from build123d import *

# Parameters (mm, degrees)
CYLINDER032_R     = 2
CYLINDER032_DEPTH = 8
CYLINDER035_R     = 2
CYLINDER035_DEPTH = 8
CYLINDER038_R     = 1.6
CYLINDER038_DEPTH = 8
CYLINDER039_R     = 1.6
CYLINDER039_DEPTH = 8
CYLINDER037_W     = 7
CYLINDER037_H     = 8
CYLINDER037_ANGLE = 90
BOX025_W          = 78
BOX025_H          = 3
BOX025_DEPTH      = 7
BOX026_W          = 40
BOX026_H          = 3
BOX026_DEPTH      = 7
CYLINDER034_R     = 5
CYLINDER034_DEPTH = 8
CYLINDER031_R     = 5
CYLINDER031_DEPTH = 8
BOX027_W          = 40
BOX027_H          = 3
BOX027_DEPTH      = 7
CYLINDER036_W     = 7
CYLINDER036_H     = 8
CYLINDER036_ANGLE = 90


with BuildPart() as cuts:
    # Cylinder032 → Cylinder032 (new body)
    with BuildSketch(Plane(origin=(13.5, -2, 61.5), x_dir=(1, 0, 0), z_dir=(0, -1, 0))):
        Circle(CYLINDER032_R)
    extrude(amount=CYLINDER032_DEPTH)


with BuildPart() as cuts001:
    # Cylinder035 → Cylinder035 (new body)
    with BuildSketch(Plane(origin=(62.5, -2, 61.5), x_dir=(1, 0, 0), z_dir=(0, -1, 0))):
        Circle(CYLINDER035_R)
    extrude(amount=CYLINDER035_DEPTH)


with BuildPart() as m3screw:
    # Cylinder038 → Cylinder038 (new body)
    with BuildSketch(Plane(origin=(75.5, -2, 100.5), x_dir=(1, 0, 0), z_dir=(0, -1, 0))):
        Circle(CYLINDER038_R)
    extrude(amount=CYLINDER038_DEPTH)


with BuildPart() as c4oldcuts:
    # Cylinder039 → Cylinder039 (new body)
    with BuildSketch(Plane(origin=(2.5, -2, 100.5), x_dir=(1, 0, 0), z_dir=(0, -1, 0))):
        Circle(CYLINDER039_R)
    extrude(amount=CYLINDER039_DEPTH)

    # Fusion016: union cuts, cuts001, m3Screw
    add(cuts.part)
    add(cuts001.part)
    add(m3screw.part)


with BuildPart() as cylinder037:
    # Cylinder037 → Cylinder037 (revolve)
    with BuildSketch(Plane(origin=(0, -2, 98), x_dir=(1, 0, 0), z_dir=(0, 0, -1))):
        with Locations((3.5, 4)):
            Rectangle(CYLINDER037_W, CYLINDER037_H)
    revolve(axis=Axis((0, -2, 98), (0, -1, 0)), revolution_arc=CYLINDER037_ANGLE)


with BuildPart() as cube020:
    # Box025 → Box025 (new body)
    with BuildSketch(Plane(origin=(0, -5, 58), x_dir=(1, 0, 0), z_dir=(0, 0, 1))):
        with Locations((39, 1.5)):
            Rectangle(BOX025_W, BOX025_H)
    extrude(amount=BOX025_DEPTH)


with BuildPart() as cube021:
    # Box026 → Box026 (new body)
    with BuildSketch(Plane(origin=(7, -5, 58), x_dir=(0, 0, 1), z_dir=(-1, 0, 0))):
        with Locations((20, 1.5)):
            Rectangle(BOX026_W, BOX026_H)
    extrude(amount=BOX026_DEPTH)


with BuildPart() as cylinder034:
    # Cylinder034 → Cylinder034 (new body)
    with BuildSketch(Plane(origin=(62.5, -2, 61.5), x_dir=(1, 0, 0), z_dir=(0, -1, 0))):
        Circle(CYLINDER034_R)
    extrude(amount=CYLINDER034_DEPTH)


with BuildPart() as cylinder031:
    # Cylinder031 → Cylinder031 (new body)
    with BuildSketch(Plane(origin=(13.5, -2, 61.5), x_dir=(1, 0, 0), z_dir=(0, -1, 0))):
        Circle(CYLINDER031_R)
    extrude(amount=CYLINDER031_DEPTH)


with BuildPart() as fusion014:
    # Box027 → Box027 (new body)
    with BuildSketch(Plane(origin=(78, -5, 58), x_dir=(0, 0, 1), z_dir=(-1, 0, 0))):
        with Locations((20, 1.5)):
            Rectangle(BOX027_W, BOX027_H)
    extrude(amount=BOX027_DEPTH)

    # Fusion014: union Cube020, Cube021, Cylinder034, Cylinder031
    add(cube020.part)
    add(cube021.part)
    add(cylinder034.part)
    add(cylinder031.part)


with BuildPart() as c4hold001:
    # Cylinder036 → Cylinder036 (revolve)
    with BuildSketch(Plane(origin=(78, -2, 98), x_dir=(0, 0, 1), z_dir=(1, 0, 0))):
        with Locations((3.5, 4)):
            Rectangle(CYLINDER036_W, CYLINDER036_H)
    revolve(axis=Axis((78, -2, 98), (0, -1, 0)), revolution_arc=CYLINDER036_ANGLE)

    # Fusion015: union Cylinder037, Fusion014
    add(cylinder037.part)
    add(fusion014.part)

    # Cut024: cut c4oldCuts
    add(c4oldcuts.part, mode=Mode.SUBTRACT)


solid = c4hold001.part
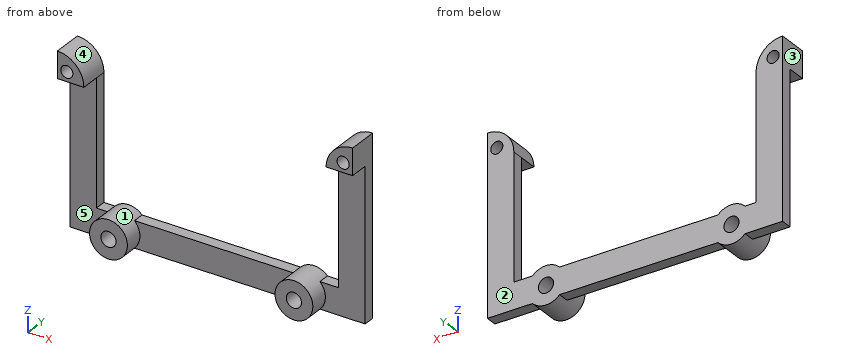
Build history of the part. All positions in model axes, mm. Face numbers are marked on the shaded views. A direction names the side the tool comes from. Give positions to 0.01 mm unless a question says otherwise; leave off trailing zeros. Write each loop counter-clockwise with the first axis right and the second up, starting at its lowest first coordinate (ties: lowest second). Pieces come first, ordered by that corner, then holes. Notation, with made-up numbers: (79, 80.25) - (102, 80.25) arc R22 ccw to (102, 86.25) - close; hole circle Ø10 at (46.25, -28.75). An arc over 180 degrees is marked (long way). Use one line per item in the form item = value. Start each with the question number.
1. Band-saw the part on B-B on x = 13.5. Write the cut outline in (y, z).
2. Probe line 1 (Z direction, x = 13.5, y = -4.25); line 2 (X direction, y = -4, z = 79); line 3 (X direction, y = -5.25, z = 100.5). List the from-to ranges inside material, lowest first. Write a range as [from, to].
3. 3-axis set-ups, long thin cutter, end or side, ignore diameter. For the marked faces 1 and 2: which of +Z, -Z, +X, -X, +Y, -Y reach the whole face in a straight line?
4. Band-saw the part on D-D on z = 61.5. Write the cut outline in (x, y), plus the area to 3 significant figures.
5. Drop flat-ended pins along their axis: pin 1 Ø5 at (x, z) = (5, 84.5) entering from -Y; pin 2 Ø4 at (x, y) = (58.5, -4) entering from +Z; pin 3 Ø2.5 at (x, y) = (69.5, -3.5) entering from +Z; pin 4 Ø4 at (x, z) = (75.5, 100.5) entering from +Y. Give the stop position or say it passes through.
6. Band-saw the part on C-C on z = 90. Write the cut outline in (x, y), plus the area to 3 significant figures.
7. Two-plate mould, pull along X, no slides. Class the marked faces 3, 4 and 5: released by +X, released by -X, zero draft, split by the parting line, or undercut.
8. Band-saw the part on A-A on y = -7.5. Write the cut outline in (x, z), plus the area to 3 significant figures.
Conclusion:
q1.outline = (-10, 56.5) - (-2, 56.5) - (-2, 59.5) - (-10, 59.5) - close; (-10, 63.5) - (-2, 63.5) - (-2, 66.5) - (-10, 66.5) - close
q2.line_1 = [56.5, 59.5], [63.5, 66.5]
q2.line_2 = [0, 7], [71, 78]
q2.line_3 = [0, 0.9], [4.1, 6.54], [71.46, 73.9], [77.1, 78]
q3.face_1 = -Y
q3.face_2 = +Z, -Z, +X, -X, +Y
q4.outline = (0, -5) - (8.5, -5) - (8.5, -10) - (11.5, -10) - (11.5, -2) - (0, -2) - close; (15.5, -10) - (18.5, -10) - (18.5, -5) - (57.5, -5) - (57.5, -10) - (60.5, -10) - (60.5, -2) - (15.5, -2) - close; (64.5, -10) - (67.5, -10) - (67.5, -5) - (78, -5) - (78, -2) - (64.5, -2) - close
q4.area = 270 mm²
q5.pin_1 = -5
q5.pin_2 = 66.08
q5.pin_3 = 65
q5.pin_4 = -2
q6.outline = (0, -5) - (7, -5) - (7, -2) - (0, -2) - close; (71, -5) - (78, -5) - (78, -2) - (71, -2) - close
q6.area = 42.0 mm²
q7.face_3 = released by -X
q7.face_4 = undercut
q7.face_5 = zero draft
q8.outline = (0, 98) - (7, 98) arc R7 ccw to (0, 105) - close; circle Ø10 at (13.5, 61.5); circle Ø10 at (62.5, 61.5); (71, 98) - (78, 98) - (78, 105) arc R7 ccw to start; hole circle Ø3.2 at (2.5, 100.5); hole circle Ø4 at (13.5, 61.5); hole circle Ø4 at (62.5, 61.5); hole circle Ø3.2 at (75.5, 100.5)
q8.area = 193 mm²
